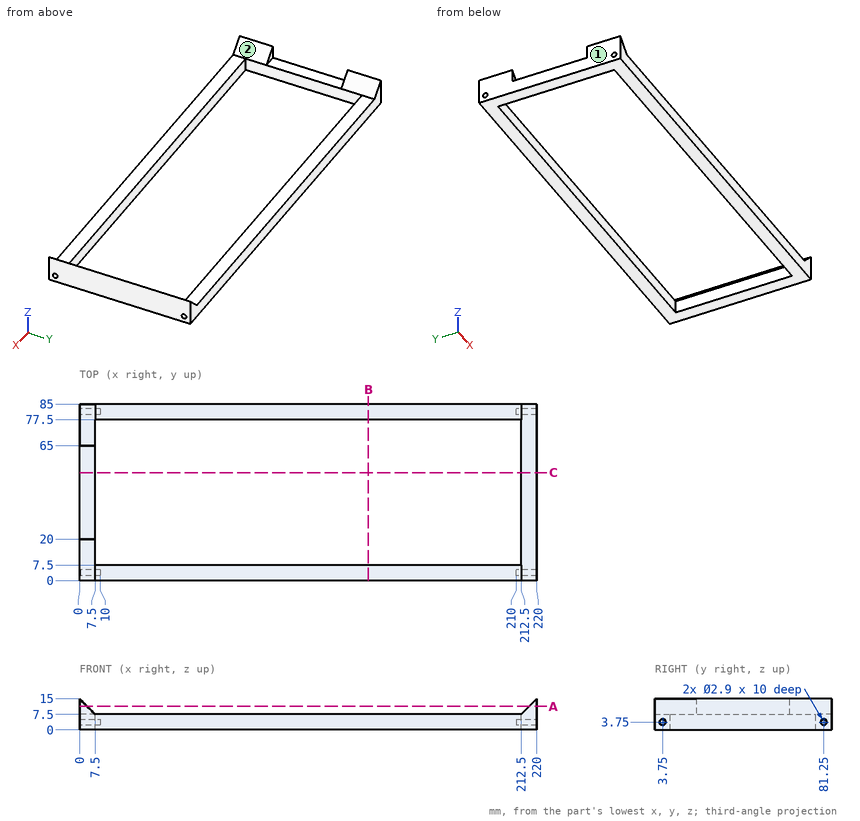
Input: dimensioned drawing with shaded views. Units: mm. Origin: part minimum x, y, z. A direction names the side the tool comes from. Give positions to 0.01 mm unless a question says otherwise; leave off trailing zeros. Write each loop counter-clockwise with the first axis right and the second up, starting at its lowest first coordinate (ties: lowest second). Pieces come first, ordered by that corner, then holes. Notation, with made-up numbers: (45.25, -12) -> (97.25, -12) arc R13 cw to (97.25, 4) -> close; hole circle Ø10 at (48.5, -10). An arc over 180 degrees is marked (long way). Return JSON: item names as keys, results as strings. Group by question number.
1. Section C-C, the plane y = 52. Output: boundary loops of the cut face in (x, z).
2. Section A-A, the plane z = 11.25. Output: boundary loops of the cut face in (x, y), then the cut area to 3 significant figures.
3. Access query for the marked faces 1 and 2. Directions: +Z, -Z, +X, -X, +Y, -Y. A direction counts if a zero-diameter tool reaches every point of the face in a straight line with its end or side. Return the directions, or none.
4. Section B-B, the plane x = 139. Output: boundary loops of the cut face in (y, z), then the cut area to 4 significant figures.
5. Material intervals for line 1 (Y direction, x = 4.25, z = 3.75); line 2 (Y direction, x = 8, z = 3.75); line 3 (X direction, y = 53.5, z = 5.75), sorted ascending. Write a range as from..to.
6. Pin query (flat end, axial travel): pin 1 Ø2.5 at (y, z) = (81.25, 3.75) entering from -X; pin 2 Ø2.5 at (y, z) = (3.75, 3.75) entering from +X; pin 3 Ø6 at (x, y) = (146, 2.5) entering from +Z. Return the tip coordinate at first contact, or that it passes through.
Determined:
{
 "1": {"outline": "(0, 0) -> (7.5, 0) -> (7.5, 7.5) -> (0, 7.5) -> close; (212.5, 0) -> (220, 0) -> (220, 15) -> (212.5, 7.5) -> close"},
 "2": {"outline": "(0, 0) -> (3.75, 0) -> (3.75, 20) -> (0, 20) -> close; (0, 65) -> (3.75, 65) -> (3.75, 85) -> (0, 85) -> close; (216.25, 0) -> (220, 0) -> (220, 85) -> (216.25, 85) -> close", "area": "469 mm2"},
 "3": {"face 1": "+Z, -Z, -X, +Y, -Y", "face 2": "+Z, +Y, -Y"},
 "4": {"outline": "(0, 0) -> (7.5, 0) -> (7.5, 7.5) -> (0, 7.5) -> close; (77.5, 0) -> (85, 0) -> (85, 7.5) -> (77.5, 7.5) -> close", "area": "112.5 mm2"},
 "5": {"line 1": "y = 0..2.3, 5.2..79.8, 82.7..85", "line 2": "y = 0..2.3, 5.2..7.5, 77.5..79.8, 82.7..85", "line 3": "x = 0..7.5, 212.5..220"},
 "6": {"pin 1": "stops at x = 10", "pin 2": "stops at x = 210", "pin 3": "stops at z = 7.5"}
}
